Verification items for the finished model (mm, model axes). Face numbers are marked on the shaded views. A direction names the side the tool comes from. Give positions to 0.01 mm unless a question says otherwise; leave off trailing zeros. Write each loop counter-clockwise with the first axis right and the second up, starting at its lowest first coordinate (ties: lowest second). Pieces come first, ordered by that corner, then holes. Notation, with made-up numbers: (17.5, 6) - (55.5, 6) arc R31 ccw to (55.5, 31) - close; hole circle Ø4 at (-38.75, -5.5). An arc over 180 degrees is marked (long way). Answer as a JSON object with one key per item and string values. Group by question number.
Item 1: Tool access check on the marked faces 3 and 4. Record the directions out of +Z, -Z, +X, -X, +Y, -Y that give a thin tool (end or side, any length) a straight path to the whole face; none if there is none.
Item 2: Scan lines: line 1 along Y through (x, z) = (16, 1); line 2 along X through (y, z) = (15.5, -3.5); line 3 along Y through (x, z) = (0, 9.75). Record each from-to range of solid material in increasing order. Write a range as [from, to].
Item 3: Draft check along X on the marked faces 1 and 2. Enter one of: +X half, -X half, draft (parallel to the pull), parting line (faces both ways), or undercut.
Item 4: Sectioned sample at B-B, the plane z = 5.5. Record the boundary of the cut face in (x, y) (3 decimals), and give its area (3 significant figures).
Item 5: Sectioned sample at C-C, the plane y = -26. Count the separate pieces of the cut face and the enclosed holes in it, and give its area (3 significant figures).
Item 6: Sectioned sample at A-A, the plane z = -1.5. Record the boundary of the cut face in (x, y) (3 decimals), and give its area (3 significant figures).
Item 7: Go/stop test with flat-tipped pins: pin 1 (8 mm diameter, centred on x = 22.5, y = -9, fed in from +Z); pin 2 (12 mm diameter, centred on y = 12, z = -7, fed in from -X); pin 3 (2 mm diameter, centred on y = -22, z = 2, fed in from -X). Record where each tip stops, or that it passes through.
```python
from build123d import *

# Parameters (mm, degrees)
ESQUISSE1_R                   = 40
BOSS_EXTRU_1_DEPTH            = 15
ESQUISSE2_R                   = 9.65
ENL_V_MAT_EXTRU_1_DEPTH       = 10.5
ENL_V_MAT_EXTRU_2_REACH       = 59.535
ESQUISSE3_R                   = 4.25
ENL_V_MAT_EXTRU_4_DEPTH       = 0.75
ENL_V_MAT_EXTRU_4_DEPTH_BACK  = 0.75
ESQUISSE4_R                   = 40
ESQUISSE4_R_2                 = 39.3
ENL_V_MAT_EXTRU_5_DEPTH       = 0.75
ENL_V_MAT_EXTRU_5_DEPTH_BACK  = 0.75
ESQUISSE5_R                   = 40
ESQUISSE5_R_2                 = 39.3
ENL_V_MAT_EXTRU_6_DEPTH       = 0.75
ENL_V_MAT_EXTRU_6_DEPTH_BACK  = 0.75
ESQUISSE6_R                   = 40
ESQUISSE6_R_2                 = 39.3
CONG_1_R                      = 5
ESQUISSE12_R                  = 35
BOSS_EXTRU_8_DEPTH            = 10
BOSS_EXTRU_2_START            = 10.5
ESQUISSE8_R                   = 9.65
BOSS_EXTRU_2_DEPTH            = 10.5
ENL_V_START                   = -25
ESQUISSE13_R                  = 4.25
ENL_V_MAT_EXTRU_10_DEPTH      = 25
ENL_V_MAT_EXTRU_11_DEPTH      = 25
ENL_V_MAT_EXTRU_12_DEPTH      = 2
ENL_V_MAT_EXTRU_12_DEPTH_BACK = 2
ESQUISSE16_R                  = 35
ESQUISSE16_R_2                = 31
CONG_2_R                      = 2


# Some blends are built 0.0001 mm under size
with BuildPart() as part:
    # Esquisse1 → Boss.-Extru.1 (new body)
    with BuildSketch(Plane.XY):
        Circle(ESQUISSE1_R)
    extrude(amount=BOSS_EXTRU_1_DEPTH)

    # Esquisse2 → Enlèv. mat.-Extru.1 (cut)
    with BuildSketch(Plane(origin=(0, 0, 0), x_dir=(-1, 0, 0), z_dir=(0, 0, -1))):
        Circle(ESQUISSE2_R)
    extrude(amount=-ENL_V_MAT_EXTRU_1_DEPTH, mode=Mode.SUBTRACT)

    # Esquisse3 → Enlèv. mat.-Extru.2 (cut, up to next)
    with BuildSketch(Plane(origin=(0, 0, 10.5), x_dir=(-1, 0, 0), z_dir=(0, 0, -1)), mode=Mode.PRIVATE) as enl_v_mat_extru_2_sk1:
        Circle(ESQUISSE3_R)
    enl_v_mat_extru_2_tool1 = extrude(enl_v_mat_extru_2_sk1.sketch, amount=-ENL_V_MAT_EXTRU_2_REACH, mode=Mode.PRIVATE) & part.part
    add(enl_v_mat_extru_2_tool1.solids().sort_by_distance((0, 0, 10.5))[0], mode=Mode.SUBTRACT)

    # Esquisse4 → Enlèv. mat.-Extru.4 (cut, two sides: drawn at the far end of the back side and taken through both)
    with BuildSketch(Plane.XY.offset(7.5).offset(-ENL_V_MAT_EXTRU_4_DEPTH_BACK)):
        Circle(ESQUISSE4_R)
        Circle(ESQUISSE4_R_2, mode=Mode.SUBTRACT)
    extrude(amount=ENL_V_MAT_EXTRU_4_DEPTH + ENL_V_MAT_EXTRU_4_DEPTH_BACK, mode=Mode.SUBTRACT)

    # Esquisse5 → Enlèv. mat.-Extru.5 (cut, two sides: drawn at the far end of the back side and taken through both)
    with BuildSketch(Plane.XY.offset(11.25).offset(-ENL_V_MAT_EXTRU_5_DEPTH_BACK)):
        Circle(ESQUISSE5_R)
        Circle(ESQUISSE5_R_2, mode=Mode.SUBTRACT)
    extrude(amount=ENL_V_MAT_EXTRU_5_DEPTH + ENL_V_MAT_EXTRU_5_DEPTH_BACK, mode=Mode.SUBTRACT)

    # Esquisse6 → Enlèv. mat.-Extru.6 (cut, two sides: drawn at the far end of the back side and taken through both)
    with BuildSketch(Plane(origin=(0, 0, 3.75), x_dir=(-1, 0, 0), z_dir=(0, 0, -1)).offset(-ENL_V_MAT_EXTRU_6_DEPTH_BACK)):
        Circle(ESQUISSE6_R)
        with Locations(Location((0, 0, 0), (0, 0, 180))):
            Circle(ESQUISSE6_R_2, mode=Mode.SUBTRACT)
    extrude(amount=ENL_V_MAT_EXTRU_6_DEPTH + ENL_V_MAT_EXTRU_6_DEPTH_BACK, mode=Mode.SUBTRACT)

    # Congé1
    # the kernel refuses this fillet: 5 mm, written as the material it takes off along each edge
    with BuildSketch(Plane(origin=(0, 0, 0), x_dir=(1, 0, 0), z_dir=(0, -1, 0))) as cong_1_piece_1:
        with BuildLine():
            CenterArc((35.417424305, 5), CONG_1_R, 270, 66.421821522)
            Line((35.417424305, 0), (35.417424305, -0.1))
            Line((35.417424305, -0.1), (40, -0.1))
            Line((40, -0.1), (40.1, 0))
            ThreePointArc((40.1, 0), (40.1, 1.5), (40.091651514, 2.96))
            Line((40.091651514, 2.96), (40, 3))
        make_face()
    revolve(axis=Axis((0, 0, 0), (0, 0, 1)), mode=Mode.SUBTRACT)
    with BuildSketch(Plane(origin=(0, 0, 15), x_dir=(1, 0, 0), z_dir=(0, -1, 0))) as cong_1_piece_2:
        with BuildLine():
            CenterArc((35.417424305, -5), CONG_1_R, 23.578178478, 66.421821522)
            Line((35.417424305, 0), (35.417424305, 0.1))
            Line((35.417424305, 0.1), (40, 0.1))
            Line((40, 0.1), (40.1, 0))
            ThreePointArc((40.1, 0), (40.1, -1.5), (40.091651514, -2.96))
            Line((40.091651514, -2.96), (40, -3))
        make_face()
    revolve(axis=Axis((0, 0, 15), (0, 0, 1)), mode=Mode.SUBTRACT)

    # Esquisse12 → Boss.-Extru.8 (add)
    with BuildSketch(Plane(origin=(0, 0, 0), x_dir=(-1, 0, 0), z_dir=(0, 0, -1))):
        with Locations(Location((0, 0, 0), (0, 0, 180))):
            Circle(ESQUISSE12_R)
    extrude(amount=BOSS_EXTRU_8_DEPTH)

    # Esquisse8 → Boss.-Extru.2 (add)
    with BuildSketch(Plane(origin=(0, 0, 10.5), x_dir=(-1, 0, 0), z_dir=(0, 0, -1)).offset(BOSS_EXTRU_2_START)):
        Circle(ESQUISSE8_R)
    extrude(amount=-BOSS_EXTRU_2_DEPTH)

    # Esquisse13 → Enlèv. mat.-Extru.10 (cut)
    with BuildSketch(Plane.XY.offset(15).offset(ENL_V_START)):
        with Locations(Location((0, 0, 0), (0, 0, 180))):
            Circle(ESQUISSE13_R)
    extrude(amount=ENL_V_MAT_EXTRU_10_DEPTH, mode=Mode.SUBTRACT)

    # Esquisse15 → Enlèv. mat.-Extru.11 (cut)
    with BuildSketch(Plane(origin=(0, 0, -10), x_dir=(-1, 0, 0), z_dir=(0, 0, -1))):
        with BuildLine():
            Line((-1.559164269, -29.959456049), (-0.519721423, -9.98648535))
            ThreePointArc((-0.519721423, -9.98648535), (-3.256100362, -9.455041535), (-5.739473718, -8.188921873))
            Line((-5.739473718, -8.188921873), (-17.218421153, -24.566765619))
            ThreePointArc((-17.218421153, -24.566765619), (-9.768301085, -28.365124606), (-1.559164269, -29.959456049))
        make_face()
        with BuildLine():
            Line((-26.725232157, -13.629452159), (-8.908410719, -4.54315072))
            ThreePointArc((-8.908410719, -4.54315072), (-9.816356344, -1.907655137), (-9.961551231, 0.876069107))
            Line((-9.961551231, 0.876069107), (-29.884653692, 2.628207322))
            ThreePointArc((-29.884653692, 2.628207322), (-29.449069033, -5.722965411), (-26.725232157, -13.629452159))
        make_face()
        with BuildLine():
            Line((-25.166067888, 16.330003891), (-8.388689296, 5.44333463))
            ThreePointArc((-8.388689296, 5.44333463), (-6.560255983, 7.547386398), (-4.222077513, 9.06499098))
            Line((-4.222077513, 9.06499098), (-12.666232538, 27.194972941))
            ThreePointArc((-12.666232538, 27.194972941), (-19.680767948, 22.642159195), (-25.166067888, 16.330003891))
        make_face()
        with BuildLine():
            Line((1.559164269, 29.959456049), (0.519721423, 9.98648535))
            ThreePointArc((0.519721423, 9.98648535), (3.256100362, 9.455041535), (5.739473718, 8.188921873))
            Line((5.739473718, 8.188921873), (17.218421153, 24.566765619))
            ThreePointArc((17.218421153, 24.566765619), (9.768301085, 28.365124606), (1.559164269, 29.959456049))
        make_face()
        with BuildLine():
            Line((26.725232157, 13.629452159), (8.908410719, 4.54315072))
            ThreePointArc((8.908410719, 4.54315072), (9.816356344, 1.907655137), (9.961551231, -0.876069107))
            Line((9.961551231, -0.876069107), (29.884653692, -2.628207322))
            ThreePointArc((29.884653692, -2.628207322), (29.449069033, 5.722965411), (26.725232157, 13.629452159))
        make_face()
        with BuildLine():
            Line((25.166067888, -16.330003891), (8.388689296, -5.44333463))
            ThreePointArc((8.388689296, -5.44333463), (6.560255983, -7.547386398), (4.222077513, -9.06499098))
            Line((4.222077513, -9.06499098), (12.666232538, -27.194972941))
            ThreePointArc((12.666232538, -27.194972941), (19.680767948, -22.642159195), (25.166067888, -16.330003891))
        make_face()
    extrude(amount=-ENL_V_MAT_EXTRU_11_DEPTH, mode=Mode.SUBTRACT)

    # Esquisse16 → Enlèv. mat.-Extru.12 (cut, two sides: drawn at the far end of the back side and taken through both)
    with BuildSketch(Plane(origin=(0, 0, -5), x_dir=(-1, 0, 0), z_dir=(0, 0, -1)).offset(-ENL_V_MAT_EXTRU_12_DEPTH_BACK)):
        with Locations(Location((0, 0, 0), (0, 0, 180))):
            Circle(ESQUISSE16_R)
        Circle(ESQUISSE16_R_2, mode=Mode.SUBTRACT)
    extrude(amount=ENL_V_MAT_EXTRU_12_DEPTH + ENL_V_MAT_EXTRU_12_DEPTH_BACK, mode=Mode.SUBTRACT)

    # Congé2
    cong_2_edges = [part.edges().sort_by_distance(p)[0] for p in [
        (31, 0, -7),
        (31, 0, -3),
    ]]
    fillet(cong_2_edges, radius=CONG_2_R - 0.0001)  # a hair under: the kernel refuses the full size


solid = part.part
```
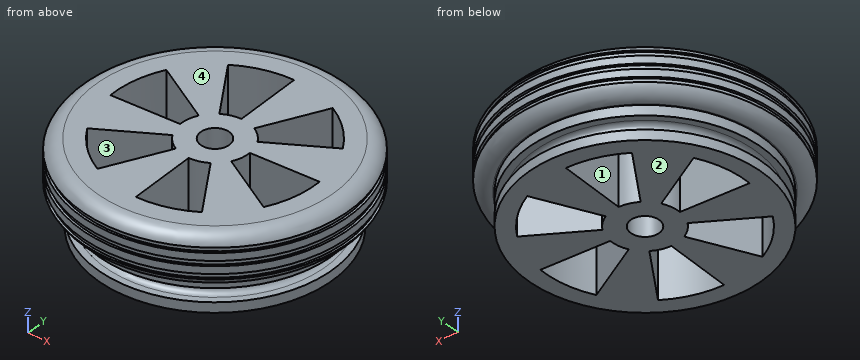
Geometry check:
{
 "1": {"face 3": "+Z, -Z", "face 4": "+Z, +X, -X, +Y, -Y"},
 "2": {"line 1": "[-34.93, -25.38], [-22.83, -8.16], [1.41, 10.38], [25.38, 34.93]", "line 2": "[-27.63, -10.86], [-0.81, 7.22], [23.89, 27.63]", "line 3": "[-40, -4.25], [4.25, 40]"},
 "3": {"face 1": "undercut", "face 2": "draft"},
 "4": {"outline": "circle Ø80 at (0, 0); hole (-29.885, -2.628) - (-9.962, -0.876) arc R10 cw to (-8.908, 4.543) - (-26.725, 13.629) arc R30 ccw to start; hole (-25.166, -16.33) arc R30 ccw to (-12.666, -27.195) - (-4.222, -9.065) arc R10 cw to (-8.389, -5.443) - close; hole (-17.218, 24.567) - (-5.739, 8.189) arc R10 cw to (-0.52, 9.986) - (-1.559, 29.959) arc R30 ccw to start; hole circle Ø8.5 at (0, 0); hole (0.52, -9.986) - (1.559, -29.959) arc R30 ccw to (17.218, -24.567) - (5.739, -8.189) arc R10 cw to start; hole (4.222, 9.065) arc R10 cw to (8.389, 5.443) - (25.166, 16.33) arc R30 ccw to (12.666, 27.195) - close; hole (8.908, -4.543) - (26.725, -13.629) arc R30 ccw to (29.885, 2.628) - (9.962, 0.876) arc R10 cw to start", "area": "3,630 mm^2"},
 "5": {"separate pieces": "3", "enclosed holes": "0", "area": "893 mm^2"},
 "6": {"outline": "circle Ø70 at (0, 0); hole (-29.885, -2.628) - (-9.962, -0.876) arc R10 cw to (-8.908, 4.543) - (-26.725, 13.629) arc R30 ccw to start; hole (-25.166, -16.33) arc R30 ccw to (-12.666, -27.195) - (-4.222, -9.065) arc R10 cw to (-8.389, -5.443) - close; hole (-17.218, 24.567) - (-5.739, 8.189) arc R10 cw to (-0.52, 9.986) - (-1.559, 29.959) arc R30 ccw to start; hole circle Ø8.5 at (0, 0); hole (0.52, -9.986) - (1.559, -29.959) arc R30 ccw to (17.218, -24.567) - (5.739, -8.189) arc R10 cw to start; hole (4.222, 9.065) arc R10 cw to (8.389, 5.443) - (25.166, 16.33) arc R30 ccw to (12.666, 27.195) - close; hole (8.908, -4.543) - (26.725, -13.629) arc R30 ccw to (29.885, 2.628) - (9.962, 0.876) arc R10 cw to start", "area": "2,450 mm^2"},
 "7": {"pin 1": "z = 15", "pin 2": "x = -34.48", "pin 3": "x = -33.7"}
}
